Autodesk Inventor part; units mm, degrees
ref_plane "YZ Plane" through (0, 0, 0) normal (1, 0, 0) x (0, 1, 0)
ref_plane "XZ Plane" through (0, 0, 0) normal (0, 1, 0) x (-1, 0, 0)
ref_plane "XY Plane" through (0, 0, 0) normal (0, 0, 1) x (1, 0, 0)
sketch "Sketch1" plane through (0, 0, 0) normal (0, 0, 1) x (1, 0, 0)
  line L0 (-20.5, -10.5) -> (20.5, -10.5)
  line L1 (20.5, -10.5) -> (20.5, 10.5)
  line L2 (20.5, 10.5) -> (-20.5, 10.5)
  line L3 (-20.5, 10.5) -> (-20.5, -10.5)
  line L4 (-20.5, -10.5) -> (20.5, 10.5) construction
  line L5 (20.5, -10.5) -> (-20.5, 10.5) construction
  circle A0 centre (25.5, 5.5) radius 1
  circle A1 centre (25.5, -5.5) radius 1
  line L6 (0, 21.6766) -> (0, -21.497) construction
  circle A2 centre (-25.5, 5.5) radius 1
  circle A3 centre (-25.5, -5.5) radius 1
  line L7 (-20.5, -10.5) -> (-30.5, -10.5)
  line L8 (-30.5, -10.5) -> (-30.5, 10.5)
  line L9 (-30.5, 10.5) -> (-20.5, 10.5)
  line L10 (-20.5, 10.5) -> (-20.5, -10.5)
  line L11 (20.5, -10.5) -> (30.5, -10.5)
  line L12 (30.5, -10.5) -> (30.5, 10.5)
  line L13 (30.5, 10.5) -> (20.5, 10.5)
  line L14 (20.5, 10.5) -> (20.5, -10.5)
  line L15 (-30.5, 10.5) -> (30.5, 10.5)
  line L16 (30.5, 10.5) -> (30.5, 15.5)
  line L17 (30.5, 15.5) -> (-30.5, 15.5)
  line L18 (-30.5, 15.5) -> (-30.5, 10.5)
  line L19 (-30.5, -10.5) -> (-40.5, -10.5)
  line L20 (-40.5, -10.5) -> (-40.5, -5.5)
  line L21 (-40.5, -5.5) -> (-30.5, -5.5)
  line L22 (-30.5, -5.5) -> (-30.5, -10.5)
  line L23 (30.5, -10.5) -> (40.5, -10.5)
  line L24 (40.5, -10.5) -> (40.5, -5.5)
  line L25 (40.5, -5.5) -> (30.5, -5.5)
  line L26 (30.5, -5.5) -> (30.5, -10.5)
  point P0 (0, 0)
  dimension "d0" = 41
  dimension "d1" = 21
  dimension "d2" = 2
  dimension "d3" = 2
  dimension "d4" = 10
  dimension "d5" = 10
  dimension "d6" = 5
  dimension "d7" = 10
  dimension "d8" = 5
  dimension "d9" = 10
extrude "Extrusion1" add sketch "Sketch1" along normal blind 15 contours L7 L8 L9 L3 | L1 L13 L12 L11 | L9 L18 L17 L16 L13 L2 | L19 L20 L21 L8 | L12 L25 L24 L23
sketch "Sketch2" plane through (30.5, -5.5, 0) normal (0, 1, 0) x (1, 0, 0)
  circle A0 centre (5, -7.5) radius 2
  point P0 (-30.5, 0)
  dimension "d12" = 4
extrude "Extrusion2" cut sketch "Sketch2" against normal through all
mirror "Mirror1" about plane through (0, 0, 0) normal (1, 0, 0) of "Extrusion2"
properties part number "PinewoodServoMount"
Verification items for the finished model (mm, model axes). A direction names the side the tool comes from. Coordinates: 2 decimals unless noted, no trailing zeros. Write each loop counter-clockwise with the first axis right and the second up, starting at its lowest first coordinate (ties: lowest second). Pieces come first, ordered by that corner, then holes. Notation, with made-up numbers: M 88,10 L 137,10 A20 cw 137,14 Z; hole C 40,26 d1. An arc over 180 degrees is marked long. Answer as a JSON object with one key per item and string values. Group by question number.
(1) Cross-section at C-C, the plane x = 35.5. Record the cut outline in (y, z), and give its area (3 significant figures).
(2) Tool access check on faces 1 (the face through (-30.5, 5, 7)), 2 (the face through (0, 10.5, 7)), 3 (the face through (25.37, -6.49, 7.4)), 4 (the face through (36.7, -5.5, 5.7)). Record the directions out of +Z, -Z, +X, -X, +Y, -Y that give a thin tool (end or side, any length) a straight path to the whole face; none if there is none.
(3) Material ranges on line 1 (X direction, y = -8.8, z = 7.5); line 2 (Y direction, x = -25.5, z = 11.25); line 3 (Z direction, x = 35.5, y = -7.2), recorded low to high.
(4) Gauge pin test, flat ends, axial feed: pin 1 (2 mm diameter, centred on x = -13.5, z = 6, fed in from -Y); pin 2 (3 mm diameter, centred on y = 6, z = 7, fed in from -X); pin 3 (4.5 mm diameter, centred on y = 5, z = 4.5, fed in from +X); pin 4 (3 mm diameter, centred on x = -25.5, y = 5.5, fed in from -Z). Record the tip position at first contact, or that the pin passes through.
(5) Cross-section at B-B, the plane y = 7.75. Record the cut outline in (x, z).
(6) Cross-section at A-A, the plane z = 7.5. Record the cut outline in (x, y).
(7) Cross-section at D-D, the plane z = 3.5. Record the cut outline in (x, y).
(8) Release check for a two-part mould opening along X. For faces 5 (the face through (-36.7, -5.5, 5.7)), 6 (the face through (-40.5, -8, 7)), 7 (the face through (-25.63, -6.49, 7.4)) record: +X half, -X half, draft (parallel to the pull), parting line (faces both ways), or undercut.
Reply:
{
 "1": {"outline": "M -10.5,0 L -5.5,0 L -5.5,5.5 L -10.5,5.5 Z; M -10.5,9.5 L -5.5,9.5 L -5.5,15 L -10.5,15 Z", "area": "55.0 mm²"},
 "2": {"face 1": "+Z, -Z, -X, +Y", "face 2": "+Z, -Z, -Y", "face 3": "+Z, -Z", "face 4": "+Z, -Z, +X, +Y"},
 "3": {"line 1": "-40.5 to -37.5, -33.5 to -20.5, 20.5 to 33.5, 37.5 to 40.5", "line 2": "-10.5 to -6.5, -4.5 to 4.5, 6.5 to 15.5", "line 3": "0 to 5.5, 9.5 to 15"},
 "4": {"pin 1": "y = 10.5", "pin 2": "x = -30.5", "pin 3": "x = 30.5", "pin 4": "z = 0"},
 "5": {"outline": "M -30.5,0 L -20.5,0 L -20.5,15 L -30.5,15 Z; M 20.5,0 L 30.5,0 L 30.5,15 L 20.5,15 Z"},
 "6": {"outline": "M -40.5,-10.5 L -37.5,-10.5 L -37.5,-5.5 L -40.5,-5.5 Z; M -33.5,-10.5 L -20.5,-10.5 L -20.5,10.5 L 20.5,10.5 L 20.5,-10.5 L 33.5,-10.5 L 33.5,-5.5 L 30.5,-5.5 L 30.5,15.5 L -30.5,15.5 L -30.5,-5.5 L -33.5,-5.5 Z; M 37.5,-10.5 L 40.5,-10.5 L 40.5,-5.5 L 37.5,-5.5 Z; hole C -25.5,-5.5 d2; hole C -25.5,5.5 d2; hole C 25.5,-5.5 d2; hole C 25.5,5.5 d2"},
 "7": {"outline": "M -40.5,-10.5 L -20.5,-10.5 L -20.5,10.5 L 20.5,10.5 L 20.5,-10.5 L 40.5,-10.5 L 40.5,-5.5 L 30.5,-5.5 L 30.5,15.5 L -30.5,15.5 L -30.5,-5.5 L -40.5,-5.5 Z; hole C -25.5,-5.5 d2; hole C -25.5,5.5 d2; hole C 25.5,-5.5 d2; hole C 25.5,5.5 d2"},
 "8": {"face 5": "draft", "face 6": "-X half", "face 7": "undercut"}
}
